Autodesk Fusion 360 part; units mm, degrees
sketch "Sketch1" plane through (0, 0, 0) normal (0, 1, 0) x (1, 0, 0)
  line L0 (0, 0) -> (47, 0)
  line L1 (47, 0) -> (47, -30)
  line L2 (47, -30) -> (0, -30)
  line L3 (0, -30) -> (0, 0)
  line L4 (47, -7.029) -> (50, -7.029)
  line L5 (50, -7.029) -> (50, -23.029)
  line L6 (50, -23.029) -> (47, -23.029)
  line L7 (47, -23.029) -> (47, -7.029)
  dimension "d1" = 47
  dimension "d2" = 30
  dimension "d3" = 16
extrude "Extrude1" add sketch "Sketch1" along normal blind 3
sketch "Sketch2" plane through (0, 3, 0) normal (0, 1, 0) x (-1, 0, 0)
  line L0 (-50, 23.029) -> (-50, 7.029)
  line L1 (-50, 7.029) -> (-47, 7.029)
  line L2 (-47, 7.029) -> (-47, 0)
  line L3 (-47, 0) -> (0, 0)
  line L4 (0, 0) -> (0, 30)
  line L5 (0, 30) -> (-47, 30)
  line L6 (-47, 30) -> (-47, 23.029)
  line L7 (-47, 23.029) -> (-50, 23.029)
  line L8 (-50, 23.029) -> (-47, 23.029)
  line L9 (-47, 23.029) -> (-47, 7.029)
  line L10 (-47, 7.029) -> (-50, 7.029)
  line L11 (-50, 7.029) -> (-50, 23.029)
  line L12 (-47, 30) -> (0, 30)
  line L13 (0, 30) -> (0, 0)
  line L14 (0, 0) -> (-47, 0)
  line L15 (-47, 0) -> (-47, 30)
  circle A0 centre (-44, 27) radius 3
  circle A1 centre (-3, 27) radius 3
  circle A2 centre (-44, 3) radius 3
  circle A3 centre (-3, 3) radius 3
  circle A4 centre (-3, 3) radius 1.5
  circle A5 centre (-44, 3) radius 1.5
  circle A6 centre (-44, 27) radius 1.5
  circle A7 centre (-3, 27) radius 1.5
  dimension "d6" = 6
  dimension "d7" = 3
  dimension "d8" = 3
  dimension "d9" = 3
extrude "Extrude2" add sketch "Sketch2" along normal blind 2 contours L5 L6 L12 L15 A0 | A0 | L2 L3 L14 L15 A2 | A2 | L4 L5 L12 L13 A1 | A1 | L3 L4 L13 L14 A3 | A3
sketch "Sketch3" plane through (0, 0, 0) normal (0, -1, 0) x (1, 0, 0)
  line L0 (50, 7.029) -> (50, 23.029)
  line L1 (50, 23.029) -> (47, 23.029)
  line L2 (47, 23.029) -> (47, 30)
  line L3 (47, 30) -> (0, 30)
  line L4 (0, 30) -> (0, 0)
  line L5 (0, 0) -> (47, 0)
  line L6 (47, 0) -> (47, 7.029)
  line L7 (47, 7.029) -> (50, 7.029)
  circle A0 centre (3, 27) radius 3
  circle A1 centre (3, 27) radius 1.5
  circle A2 centre (44, 27) radius 3
  circle A3 centre (44, 27) radius 1.5
  circle A4 centre (3, 3) radius 3
  circle A5 centre (3, 3) radius 1.5
  circle A6 centre (44, 3) radius 3
  circle A7 centre (44, 3) radius 1.5
  dimension "d12" = 6
  dimension "d13" = 3
  dimension "d14" = 6
  dimension "d15" = 3
extrude "Extrude3" cut sketch "Sketch3" against normal blind 6 contours A1 | A3 | A5 | A7
chamfer "Chamfer1" distance 1 angle 45 1 edges at (1.6015, 0, 3.5424)
chamfer "Chamfer2" distance 1 angle 45 1 edges at (42.6015, 0, 3.5424)
chamfer "Chamfer3" distance 1 angle 45 1 edges at (1.6015, 0, 27.5424)
chamfer "Chamfer4" distance 1 angle 45 1 edges at (42.6015, 0, 27.5424)
For this review, take the finished solid that the model builds, in its own axes (mm). A direction names the side the tool comes from. Round coordinates to 2 decimals unless told otherwise and drop trailing zeros. Order: outer loops, then holes, each group sorted by start corner. A loop starts at its lowest first (then second) coordinate and runs counter-clockwise, first axis right, second up. Notation, with made-up numbers: M 16,67.25 L 25,67.25 A21 ccw 25,83.25 Z; hole C 28.25,-12 d4. An arc over 180 degrees is marked long. Write each question's results on one line, items separated by ' | '. Start each with the question number.
1. Add section C-C (z = 20.75). State the section outline as (x, y) points, then the cut area to 3 significant figures.
2. Add section B-B (x = 18.5). State the section outline as (y, z) points, then the cut area to 3 significant figures.
3. Add section A-A (y = 0.5). State the section outline as (x, z) points, then the cut area to 3 significant figures.
4. Clearance check with flat-ended pins moving along their axes: pin 1 Ø2.5 at (y, z) = (2.5, 25.5) entering from +X; pin 2 Ø0.9 at (x, y) = (49, 1) entering from -Z; pin 3 Ø6 at (x, z) = (25.5, 19.5) entering from +Y. State where each tip first meets the part, or that it passes through.
5. To check wall thickness, follow L1, parallel to Z at x = 44, y = 2; L2, parallel to Z at x = 44, y = 3.4; L3, parallel to X at y = 3.15, z = 3. State the ranges of each line that lie inside material, in increasing order. Write a range as [from, to].
6. Draft analysis for pull direction X (two halves, no side actions). For faces 4 (the face through (50, 1, 15)), 5 (the face through (23, 2, 0)), 6 (the face through (2.805, 2.972, 28.487)), state which applies: pulls with the +X half, pulls with the -X half, needs draft (parallel to the pull), parting line crosses it, or undercut.
7. Tool access review of faces 1 (the face through (1.7, 5, 1.7)), 2 (the face through (48, 1, 7.029)), 3 (the face through (41.81, 3.99, 24.95)): name each direction out of +Z, -Z, +X, -X, +Y, -Y from which nothing blocks a thin tool from reaching the whole face with its end or side.
Output values:
1) outline: M 0,0 L 50,0 L 50,3 L 0,3 Z | area: 150 mm^2
2) outline: M 0,0 L 3,0 L 3,30 L 0,30 Z | area: 90.0 mm^2
3) outline: M 0,0 L 47,0 L 47,7.03 L 50,7.03 L 50,23.03 L 47,23.03 L 47,30 L 0,30 Z; hole C 3,3 d4; hole C 3,27 d4; hole C 44,3 d4; hole C 44,27 d4 | area: 1,410 mm^2
4) pin 1: x = 47 | pin 2: z = 7.03 | pin 3: y = 3
5) L1: [0, 1.5], [4.5, 25.5], [28.5, 30] | L2: [0, 1.5], [4.5, 6], [24, 25.5], [28.5, 30] | L3: [0, 1.5], [4.5, 6], [41, 42.5], [45.5, 47]
6) face 4: pulls with the +X half | face 5: needs draft | face 6: undercut
7) face 1: +Z, -Z, +X, -X, +Y | face 2: -Z, +X, +Y, -Y | face 3: +Y
